Can you work these out from the model? Positions are in its coordinate system, mm. Round coordinates to 2 decimals unless told otherwise and drop trailing zeros. Write each loop counter-clockwise with the first axis right and the second up, starting at its lowest first coordinate (ties: lowest second). Pieces come first, ordered by that corner, then holes. Notation, with made-up numbers: M 51.25,-17.5 L 58.25,-17.5 A34 cw 58.25,21.5 Z; hole C 31.25,-2 d6. An arc over 180 degrees is marked long. Answer in a Markdown table with one row per item. Add a question column.
(1) Suppose I cut it at C-C, the plane z = 3. Write out the boundary of the cut face in (x, y).
(2) Suppose I cut it at B-B, the plane x = 0. Write out the boundary of the cut face in (y, z), then the cut area to 3 significant figures.
(3) If I drill on probe 1 along X at (y, z) = (0.8, 1.75); probe 2 along X at (y, z) = (1.75, -0.75); probe 3 along Z at (x, y) = (3, 1.5), over which ranges is the centre line in solid material (lowest first)?
(4) If we mould it in two halves opening along Z, with no side actions, what happens to faces 1 (the face through (-3.44, 2.46, -4.48)), 2 (the face through (-8.266, 2.465, 4.684)), 3 (the face through (5, 5, -4)), 4 (the face through (-8.2, 2.5, -4.8))? For each: released by +Z, released by -Z, zero draft, split by the parting line, or undercut.
(5) I'm going to push a flat-ended pin straight in: pin 1 (1.5 mm diameter, centred on y = 2, z = -3.5, fed in from -X). Where does the tip first touch, or does it pass through?
(6) Suppose I cut it at A-A, the plane y = 2.8. Write out the boundary of the cut face in (x, z), then the cut area to 3 significant figures.
(7) Suppose I cut it at D-D, the plane z = 6.5. Write out the boundary of the cut face in (x, y), then the cut area to 3 significant figures.
from build123d import *

# Parameters (mm, degrees)
ESQUISSE1_R      = 5.65
EXTRUSION1_DEPTH = 5


with BuildPart() as part:
    # Esquisse1 → Extrusion1 (new body)
    with BuildSketch(Plane(origin=(0, 0, 0), x_dir=(1, 0, 0), z_dir=(0, 1, 0))):
        Polygon((5.484827557, -9.5), (10.969655115, 0), (5.484827557, 9.5), (-5.484827557, 9.5), (-10.969655115, 0), (-5.484827557, -9.5), align=None)
        with Locations(Location((0, 0, 0), (0, 0, 270))):
            Circle(ESQUISSE1_R, mode=Mode.SUBTRACT)
    extrude(amount=EXTRUSION1_DEPTH)


solid = part.part
Calculated:
| question | item | result |
|---|---|---|
| 1 | outline | M -9.24,0 L -4.79,0 L -4.79,5 L -9.24,5 Z; M 4.79,0 L 9.24,0 L 9.24,5 L 4.79,5 Z |
| 2 | outline | M 0,-9.5 L 5,-9.5 L 5,-5.65 L 0,-5.65 Z; M 0,5.65 L 5,5.65 L 5,9.5 L 0,9.5 Z |
| 2 | area | 38.5 mm² |
| 3 | probe 1 | -9.96 to -5.37, 5.37 to 9.96 |
| 3 | probe 2 | -10.54 to -5.6, 5.6 to 10.54 |
| 3 | probe 3 | -9.5 to -4.79, 4.79 to 9.5 |
| 4 | face 1 | undercut |
| 4 | face 2 | released by +Z |
| 4 | face 3 | zero draft |
| 4 | face 4 | released by -Z |
| 5 | pin 1 | x = -9.38 |
| 6 | outline | M -10.97,0 L -5.48,-9.5 L 5.48,-9.5 L 10.97,0 L 5.48,9.5 L -5.48,9.5 Z; hole C 0,0 d11.3 |
| 6 | area | 212 mm² |
| 7 | outline | M -7.22,0 L 7.22,0 L 7.22,5 L -7.22,5 Z |
| 7 | area | 72.2 mm² |
